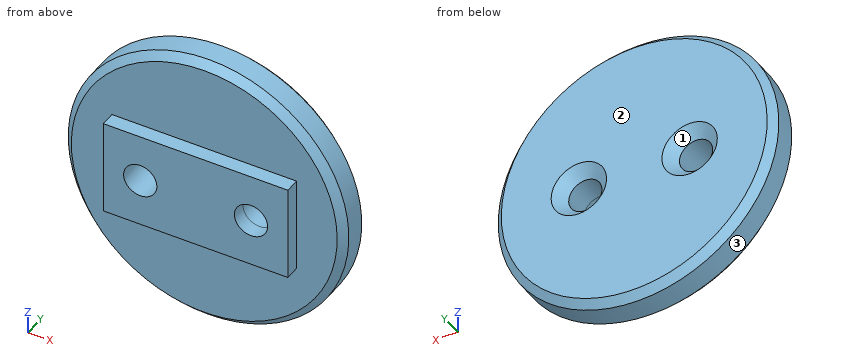
```python
from build123d import *

# Parameters (mm, degrees)
SKETCH1_R           = 19
BOSS_EXTRUDE1_DEPTH = 5
CHAMFER2_SIZE       = 1
SKETCH2_R           = 2.25
CUT_EXTRUDE1_DEPTH  = 28.331300737
CHAMFER1_SIZE       = 1.5
SKETCH3_W           = 25
SKETCH3_H           = 13
BOSS_EXTRUDE2_DEPTH = 2
SKETCH4_R           = 2.25
CUT_EXTRUDE2_DEPTH  = 28.331300737


with BuildPart() as part:
    # Sketch1 → Boss-Extrude1 (new body)
    with BuildSketch(Plane(origin=(0, 0, 0), x_dir=(1, 0, 0), z_dir=(0, 1, 0))):
        with Locations(Location((0, 0, 0), (0, 0, 270))):
            Circle(SKETCH1_R)
    extrude(amount=BOSS_EXTRUDE1_DEPTH)

    # Chamfer2
    chamfer2_edges = [part.edges().sort_by_distance(p)[0] for p in [
        (0, 0, -19),
        (0, 5, -19),
    ]]
    chamfer(chamfer2_edges, length=CHAMFER2_SIZE)

    # Sketch2 → Cut-Extrude1 (cut, through all)
    with BuildSketch(Plane(origin=(0, 5, 0), x_dir=(1, 0, 0), z_dir=(0, 1, 0))):
        with Locations(Location((-7.5, 0, 0), (0, 0, 270))):
            Circle(SKETCH2_R)
        with Locations(Location((7.5, 0, 0), (0, 0, 90))):
            Circle(SKETCH2_R)
    extrude(amount=-CUT_EXTRUDE1_DEPTH, mode=Mode.SUBTRACT)

    # Chamfer1
    chamfer1_edges = [part.edges().sort_by_distance(p)[0] for p in [
        (-7.5, 5, -2.25),
        (7.5, 5, 2.25),
    ]]
    chamfer(chamfer1_edges, length=CHAMFER1_SIZE)

    # Sketch3 → Boss-Extrude2 (add)
    with BuildSketch(Plane.XZ):
        Rectangle(SKETCH3_W, SKETCH3_H)
    extrude(amount=BOSS_EXTRUDE2_DEPTH)

    # Sketch4 → Cut-Extrude2 (cut, through all)
    with BuildSketch(Plane(origin=(0, 0, 0), x_dir=(1, 0, 0), z_dir=(0, 1, 0))):
        with Locations(Location((7.5, 0, 0), (0, 0, 270))):
            Circle(SKETCH4_R)
        with Locations(Location((-7.5, 0, 0), (0, 0, 270))):
            Circle(SKETCH4_R)
    extrude(amount=-CUT_EXTRUDE2_DEPTH, mode=Mode.SUBTRACT)


solid = part.part
```
Source: CAD feature listing. Evaluate the final solid. Frame: model axes, mm. Face numbers are marked on the shaded views. Give positions to 0.01 mm unless a question says otherwise; leave off trailing zeros. Order: outer loops, then holes, each group sorted by start corner. A loop starts at its lowest first (then second) coordinate and runs counter-clockwise, first axis right, second up.
(1) Material intervals for line 1 along X through (y, z) = (2, 0); line 2 along X through (y, z) = (-1.45, 0); line 3 along Y through (x, z) = (-12, 10), sorted ascending.
(2) Contact query for flat-ended pins moving along their axis: P1, Ø4, axis at x = -2.5, y = 3, coming from the +Z side; P2, Ø3.5, axis at x = 7.5, z = 0, coming from the +Y side; P3, Ø1, axis at x = 6, y = -1, coming from the -Z side; P4, Ø2, axis at y = -1.5, z = -2.5, coming from the +X side. Output: stop coordinate, or through.
(3) Section query B-B (x = 0). Return the cut outline in (y, z).
(4) Pull-direction query (X, two-part tool) for the marked faces 1, 2 and 3; classes: +X half, -X half, draft (parallel to the pull), parting line (faces both ways), or undercut.
(5) Section query A-A (z = 0). Return the cut outline in (x, y), plus the area to 4 significant figures.
Outcome:
1. line 1: x = -19 to -9.75, -5.25 to 5.25, 9.75 to 19
1. line 2: x = -12.5 to -9.75, -5.25 to 5.25, 9.75 to 12.5
1. line 3: y = 0 to 5
2. P1: stops at z = 18.99
2. P2: passes through
2. P3: stops at z = -6.5
2. P4: stops at x = 12.5
3. outline: (-2, -6.5) - (0, -6.5) - (0, -18) - (1, -19) - (4, -19) - (5, -18) - (5, 18) - (4, 19) - (1, 19) - (0, 18) - (0, 6.5) - (-2, 6.5) - close
4. face 1: undercut
4. face 2: draft
4. face 3: parting line
5. outline: (-19, 1) - (-18, 0) - (-12.5, 0) - (-12.5, -2) - (-9.75, -2) - (-9.75, 3.5) - (-11.25, 5) - (-18, 5) - (-19, 4) - close; (-5.25, -2) - (5.25, -2) - (5.25, 3.5) - (3.75, 5) - (-3.75, 5) - (-5.25, 3.5) - close; (9.75, -2) - (12.5, -2) - (12.5, 0) - (18, 0) - (19, 1) - (19, 4) - (18, 5) - (11.25, 5) - (9.75, 3.5) - close
5. area: 170.5 mm2
